Here's how the part is built. I have some questions about the finished solid (model axes, mm). A direction names the side the tool comes from. Coordinates: 2 decimals unless noted, no trailing zeros. Write each loop counter-clockwise with the first axis right and the second up, starting at its lowest first coordinate (ties: lowest second). Pieces come first, ordered by that corner, then holes. Notation, with made-up numbers: (-18, -6.5) -> (-14, -6.5) arc R20 cw to (-14, 28.5) -> close; hole circle Ø10 at (28.5, -31). An arc over 180 degrees is marked (long way). Use a Markdown table: item, result. Add a question column.
```python
from build123d import *

# Parameters (mm, degrees)
F0_W        = 76.2
F0_H        = 152.4
F1_DEPTH    = 6.35
F2_DEPTH    = 25.4
F0_W_2      = 31.75
F0_H_2      = 31.75
F3_DEPTH    = 50.8
F4_C1_SIZE2 = 12.7
F4_C1_SIZE  = 7.3323484187
F4_C2_SIZE2 = 12.7
F4_C2_SIZE  = 7.3323484187
F4_C3_SIZE2 = 7.3323484187
F4_C3_SIZE  = 12.7
F4_C4_SIZE2 = 12.7
F4_C4_SIZE  = 7.3323484187
F4_C5_SIZE2 = 7.3323484187
F4_C5_SIZE  = 12.7
F4_C6_SIZE2 = 7.3323484187
F4_C6_SIZE  = 12.7
F4_C7_SIZE2 = 7.3323484187
F4_C7_SIZE  = 12.7
F4_C8_SIZE2 = 12.7
F4_C8_SIZE  = 7.3323484187
F5_R        = 6.35
F6_R        = 5.08


with BuildPart() as f1:
    # F0 (on Top) → F1 (new body)
    with BuildSketch(Plane.XY):
        with Locations((2.3026284762, 11.2662552908)):
            Rectangle(F0_W, F0_H)
        Polygon((-29.4473715238, 49.3662552908), (-29.4473715238, 81.1162552908), (2.3026284762, 81.1162552908), (34.0526284762, 81.1162552908), (34.0526284762, -26.8337447092), (34.0526284762, -58.5837447092), (2.3026284762, -58.5837447092), (-29.4473715238, -58.5837447092), align=None, mode=Mode.SUBTRACT)
    extrude(amount=F1_DEPTH)

    # F0 (on Top) → F2 (join)
    with BuildSketch(Plane.XY):
        Polygon((34.0526284762, 81.1162552908), (2.3026284762, 81.1162552908), (2.3026284762, 49.3662552908), (-29.4473715238, 49.3662552908), (-29.4473715238, -58.5837447092), (2.3026284762, -58.5837447092), (2.3026284762, -26.8337447092), (34.0526284762, -26.8337447092), align=None)
    extrude(amount=F2_DEPTH)

    # F0 (on Top) → F3 (join)
    with BuildSketch(Plane.XY):
        with Locations((-13.5723715238, 65.2412552908)):
            Rectangle(F0_W_2, F0_H_2)
        with Locations((18.1776284762, -42.7087447092)):
            Rectangle(F0_W_2, F0_H_2)
    extrude(amount=F3_DEPTH)

    # F4: chamfer of 12.7 x 7.3323484187 on 8 edges, made by hand

    # F4_c1
    f4_c1_edges = [f1.edges().sort_by_distance(p)[0] for p in [
        (-13.5723715238, -58.5837447092, 25.4),
    ]]
    f4_c1_side = f1.faces().sort_by_distance((-13.5723715238, -58.5837447092, 25.2533530316))[0]
    chamfer(f4_c1_edges, length=F4_C1_SIZE, length2=F4_C1_SIZE2, reference=f4_c1_side)

    # F4_c2
    f4_c2_edges = [f1.edges().sort_by_distance(p)[0] for p in [
        (18.1776284762, -58.5837447092, 50.8),
    ]]
    f4_c2_side = f1.faces().sort_by_distance((18.1776284762, -58.5837447092, 50.6533530316))[0]
    chamfer(f4_c2_edges, length=F4_C2_SIZE, length2=F4_C2_SIZE2, reference=f4_c2_side)

    # F4_c3
    f4_c3_edges = [f1.edges().sort_by_distance(p)[0] for p in [
        (34.0526284762, -36.3587447092, 50.8),
    ]]
    f4_c3_side = f1.faces().sort_by_distance((34.0526284762, -36.3587447092, 50.6533530316))[0]
    chamfer(f4_c3_edges, length=F4_C3_SIZE, length2=F4_C3_SIZE2, reference=f4_c3_side)

    # F4_c4
    f4_c4_edges = [f1.edges().sort_by_distance(p)[0] for p in [
        (18.1776284762, 81.1162552908, 25.4),
    ]]
    f4_c4_side = f1.faces().sort_by_distance((18.1776284762, 81.1162552908, 25.2533530316))[0]
    chamfer(f4_c4_edges, length=F4_C4_SIZE, length2=F4_C4_SIZE2, reference=f4_c4_side)

    # F4_c5
    f4_c5_edges = [f1.edges().sort_by_distance(p)[0] for p in [
        (-29.4473715238, 1.7412552908, 25.4),
    ]]
    f4_c5_side = f1.faces().sort_by_distance((-29.3007245555, 1.7412552908, 25.4))[0]
    chamfer(f4_c5_edges, length=F4_C5_SIZE, length2=F4_C5_SIZE2, reference=f4_c5_side)

    # F4_c6
    f4_c6_edges = [f1.edges().sort_by_distance(p)[0] for p in [
        (34.0526284762, 20.7912552908, 25.4),
    ]]
    f4_c6_side = f1.faces().sort_by_distance((33.9059815078, 20.7912552908, 25.4))[0]
    chamfer(f4_c6_edges, length=F4_C6_SIZE, length2=F4_C6_SIZE2, reference=f4_c6_side)

    # F4_c7
    f4_c7_edges = [f1.edges().sort_by_distance(p)[0] for p in [
        (-29.4473715238, 65.2412552908, 50.8),
    ]]
    f4_c7_side = f1.faces().sort_by_distance((-29.3007245555, 65.2412552908, 50.8))[0]
    chamfer(f4_c7_edges, length=F4_C7_SIZE, length2=F4_C7_SIZE2, reference=f4_c7_side)

    # F4_c8
    f4_c8_edges = [f1.edges().sort_by_distance(p)[0] for p in [
        (-7.2223715238, 81.1162552908, 50.8),
    ]]
    f4_c8_side = f1.faces().sort_by_distance((-7.2223715238, 80.9696083224, 50.8))[0]
    chamfer(f4_c8_edges, length=F4_C8_SIZE, length2=F4_C8_SIZE2, reference=f4_c8_side)

    # F5
    f5_edges = [f1.edges().sort_by_distance(p)[0] for p in [
        (2.302628, 49.366255, 38.1),
        (2.302628, -26.833745, 38.1),
    ]]
    fillet(f5_edges, radius=F5_R)

    # F6
    f6_edges = [f1.edges().sort_by_distance(p)[0] for p in [
        (2.302628, 87.466255, 6.35),
        (40.402628, 11.266255, 6.35),
    ]]
    fillet(f6_edges, radius=F6_R)


solid = f1.part
```
Q1. Will these pins go through, and if not, where does the flat tip stop? pin 1 (9.5 mm diameter, centred on x = -11.5, z = 22.5, fed in from +Y); pin 2 (7.5 mm diameter, centred on y = -42, z = 36, fed in from -X); pin 3 (16 mm diameter, centred on y = 11.5, z = 17.5, fed in from +X).
Q2. Suppose I cut it at C-C, the plane x = -20.5. Write out the boundary of the cut face in (y, z), and give its area (3 significant figures).
Q3. Suppose I cut it at B-B, the plane y = 61.5. Write out the boundary of the cut face in (x, z), and give its area (3 significant figures).
Q4. Please list where these lines run through material, in increasing order: line 1 (Z direction, x = 35.5, y = 68.5); line 2 (Y direction, x = 31.5, z = 10); line 3 (X direction, y = 12, z = 10).
Q5. Which directions (+Z, -Z, +X, -X, +Y, -Y) give clear straight access to the entire face, cutting with the end or side of a thin tool? Please do faces 1 (the flat face through (-23.19, 63.49, 47.08)), 2 (the flat face through (2.303, -46, 38)), 3 (the flat face through (-5, 81.116, 18)), 4 (the flat face through (27.792, 26.386, 21.682)), 5 (the flat face through (14, -36, 50.8)).
Q6. Suppose I cut it at D-D, the plane z = 42. Write out the boundary of the cut face in (x, y).
Q7. Suppose I cut it at A-A, the plane z = 27. Write out the boundary of the cut face in (x, y).
Answer key:
| question | item | result |
|---|---|---|
| 1 | pin 1 | stops at y = 81.12 |
| 1 | pin 2 | stops at x = 2.3 |
| 1 | pin 3 | stops at x = 34.05 |
| 2 | outline | (-64.93, 0) -> (87.47, 0) -> (87.47, 1.27) arc R5.08 ccw to (82.39, 6.35) -> (81.12, 6.35) -> (81.12, 38.1) -> (75.03, 48.63) -> (49.37, 48.63) -> (49.37, 23.23) -> (-49.64, 23.23) -> (-58.58, 18.07) -> (-58.58, 6.35) -> (-64.93, 6.35) -> close |
| 2 | area | 4,070 mm^2 |
| 3 | outline | (-35.8, 0) -> (40.4, 0) -> (40.4, 1.27) arc R5.08 ccw to (35.32, 6.35) -> (34.05, 6.35) -> (34.05, 18.07) -> (21.35, 25.4) -> (2.3, 25.4) -> (2.3, 50.8) -> (-16.75, 50.8) -> (-29.45, 43.47) -> (-29.45, 6.35) -> (-35.8, 6.35) -> close |
| 3 | area | 2,400 mm^2 |
| 4 | line 1 | z = 0 to 6.35 |
| 4 | line 2 | y = -58.58 to 81.12 |
| 4 | line 3 | x = -29.45 to 34.05 |
| 5 | face 1 | +Z, -X, +Y, -Y |
| 5 | face 2 | +Z, -X, -Y |
| 5 | face 3 | +Z, +X, -X, +Y |
| 5 | face 4 | +Z, +X, +Y |
| 5 | face 5 | +Z, +X, -X, +Y, -Y |
| 6 | outline | (-29.45, 49.37) -> (-4.05, 49.37) arc R6.35 ccw to (2.3, 55.72) -> (2.3, 78.86) -> (-29.45, 78.86) -> close; (2.3, -58.58) -> (31.8, -58.58) -> (31.8, -26.83) -> (8.65, -26.83) arc R6.35 ccw to (2.3, -33.18) -> close |
| 7 | outline | (-29.45, 49.37) -> (-4.05, 49.37) arc R6.35 ccw to (2.3, 55.72) -> (2.3, 81.12) -> (-29.45, 81.12) -> close; (2.3, -58.58) -> (34.05, -58.58) -> (34.05, -26.83) -> (8.65, -26.83) arc R6.35 ccw to (2.3, -33.18) -> close |
